```python
from build123d import *

# Parameters (mm, degrees)
SKETCH1_R           = 22.225
BOSS_EXTRUDE1_DEPTH = 34.925
BOSS_EXTRUDE2_START = -34.925
BOSS_EXTRUDE2_DEPTH = 12.7
SKETCH2_3_W         = 304.8
SKETCH2_3_H         = 88.9
BOSS_EXTRUDE3_DEPTH = 47.625
SKETCH3_W           = 75.25
SKETCH3_H           = 68.9
CUT_EXTRUDE1_DEPTH  = 149.86


with BuildPart() as part:
    # Sketch1 → Boss-Extrude1 (new, symmetric)
    with BuildSketch(Plane(origin=(0, 0, 0), x_dir=(0, 0, -1), z_dir=(1, 0, 0))):
        Circle(SKETCH1_R)
    extrude(amount=BOSS_EXTRUDE1_DEPTH, both=True)

    # Sketch2 → Boss-Extrude2 (add)
    with BuildSketch(Plane(origin=(0, 0, 0), x_dir=(0, 0, -1), z_dir=(1, 0, 0)).offset(BOSS_EXTRUDE2_START)):
        with BuildLine():
            Line((0, 44.45), (-44.45, 44.45))
            Line((-44.45, 44.45), (-44.45, -44.45))
            Line((-44.45, -44.45), (0, -44.45))
            ThreePointArc((0, -44.45), (44.45, 0), (0, 44.45))
        make_face()
    extrude(amount=-BOSS_EXTRUDE2_DEPTH)

    # Sketch2<3> → Boss-Extrude3 (add)
    with BuildSketch(Plane(origin=(0, 0, 0), x_dir=(0, 0, -1), z_dir=(1, 0, 0))):
        with Locations((-196.85, 0)):
            Rectangle(SKETCH2_3_W, SKETCH2_3_H)
    extrude(amount=-BOSS_EXTRUDE3_DEPTH)

    # Mirror6: part across plane


with BuildPart() as part_1:
    add(part.part)
    add(part.part.mirror(Plane(origin=(0, 0, 0), x_dir=(0, 0, 1), z_dir=(1, 0, 0))))

    # Sketch3 → Cut-Extrude1 (cut)
    with BuildSketch(Plane.XY.offset(349.25)):
        Rectangle(SKETCH3_W, SKETCH3_H)
    extrude(amount=-CUT_EXTRUDE1_DEPTH, mode=Mode.SUBTRACT)


solid = part_1.part
```
Can you work these out from the model? Positions are in its coordinate system, mm. A direction names the side the tool comes from. Round coordinates to 2 decimals unless told otherwise and drop trailing zeros. Loops run counter-clockwise (first coordinate to the right, second up) from the corner with the lowest first, then second, coordinate; pieces in that order, holes last. Notation, with made-up numbers: M -34,4.5 L 22,4.5 A28 ccw 22,26.5 Z; hole C -3,80 d6. An arc over 180 degrees is marked long. Answer as a JSON object with one key per item and string values. Group by question number.
Q1. Imagine slicing it at C-C, the plane y = 0. Please give me the cut outline in (x, z) (3 decimals).
Q2. On a 3-axis mill with a long thin cutter (end or side, diameter ignored), from which of +Z, -Z, +X, -X, +Y, -Y can I reach the whole of each face in a straight line? I mean faces 1 (the flat face through (47.625, 1, 155)), 2 (the flat face through (-1, 39, 349.25)), 3 (the flat face through (0, -1, 44.45)), 4 (the flat face through (34.925, 11, 20)), 5 (the flat face through (-1, -34.45, 275)). Say none if no direction works.
Q3. Imagine slicing it at A-A, the plane x = -28. Please give me the cut outline in (y, z) (3 decimals), then the cut area to 3 significant figures.
Q4. Imagine slicing it at B-B, the plane z = 283.5. Please give me the cut outline in (x, y) (3 decimals).
Q5. Will these pins go through, and if not, where does the flat tip stop? pin 1 (6 mm diameter, centred on x = -14.5, y = 22, fed in from -Z); pin 2 (6 mm diameter, centred on x = -32, y = 18, fed in from +Z); pin 3 (4 mm diameter, centred on x = -38, y = -28.5, fed in from -Z).
Q6. Imagine slicing it at D-D, the plane z = 38. Please give me the cut outline in (x, y) (3 decimals).
Q7. Please list where these lines run through material, in increasing order: L1, parallel to X at y = 4, z = 325 (3 decimals); L2, parallel to Y at x = 10, z = 314; L3, parallel to Z at x = -8.5, y = 35.
Q8. We'd pull the mould along X, two halves only. Please class faces 6 (the flat face through (-37.625, 0, 275)), 7 (the cylindrical face through (-41.19, -0.98, -44.44)), 8 (the flat face through (-47.625, 1, 155)): +X half, -X half, draft (parallel to the pull), parting line (faces both ways), or undercut.
Findings:
{
 "1": {"outline": "M -47.625,-44.45 L -34.925,-44.45 L -34.925,-22.225 L 34.925,-22.225 L 34.925,-44.45 L 47.625,-44.45 L 47.625,349.25 L 37.625,349.25 L 37.625,199.39 L -37.625,199.39 L -37.625,349.25 L -47.625,349.25 Z; hole M -34.925,22.225 L 34.925,22.225 L 34.925,44.45 L -34.925,44.45 Z"},
 "2": {"face 1": "+Z, -Z, +X, +Y, -Y", "face 2": "+Z, +X, -X, +Y, -Y", "face 3": "+Y, -Y", "face 4": "none", "face 5": "+Z"},
 "3": {"outline": "M -44.45,44.45 L 44.45,44.45 L 44.45,349.25 L 34.45,349.25 L 34.45,199.39 L -34.45,199.39 L -34.45,349.25 L -44.45,349.25 Z; C 0,0 d44.45", "area": "18,300 mm2"},
 "4": {"outline": "M -47.625,-44.45 L 47.625,-44.45 L 47.625,44.45 L -47.625,44.45 Z; hole M -37.625,-34.45 L 37.625,-34.45 L 37.625,34.45 L -37.625,34.45 Z"},
 "5": {"pin 1": "stops at z = -11.53", "pin 2": "stops at z = 199.39", "pin 3": "stops at z = -35.69"},
 "6": {"outline": "M -47.625,-44.45 L -34.925,-44.45 L -34.925,44.45 L -47.625,44.45 Z; M 34.925,-44.45 L 47.625,-44.45 L 47.625,44.45 L 34.925,44.45 Z"},
 "7": {"L1": "x = -47.625 to -37.625, 37.625 to 47.625", "L2": "y = -44.45 to -34.45, 34.45 to 44.45", "L3": "z = 44.45 to 349.25"},
 "8": {"face 6": "undercut", "face 7": "draft", "face 8": "-X half"}
}
